Read the model definition and answer for the solid it produces. Units are mm, in the model's axes. A direction names the side the tool comes from. Give positions to 0.01 mm unless a question says otherwise; leave off trailing zeros. Loops run counter-clockwise (first coordinate to the right, second up) from the corner with the lowest first, then second, coordinate; pieces in that order, holes last. Notation, with made-up numbers: (61, 14) - (113, 14) arc R25 ccw to (113, 42) - close; hole circle Ø9 at (38, -8). An arc over 180 degrees is marked (long way). Write item = value, one per line. Start each with the question number.
from build123d import *

# Parameters (mm, degrees)
F1_DEPTH = 13.97
F3_D     = 4.7625
F4_W     = 19.05
F4_H     = 13.97
F5_DEPTH = 8.89
F7_D     = 4.7625


with BuildPart() as f1:
    # F0 (on Top) → F1 (new body)
    with BuildSketch(Plane.XY):
        with BuildLine():
            ThreePointArc((-30.457825, -6.426635), (-18.69401, -17.139455), (-7.62, -5.715))
            ThreePointArc((-7.62, -5.715), (-10.967769, 2.367231), (-19.05, 5.715))
            ThreePointArc((-19.05, 5.715), (-24.765, 4.18367), (-28.94867, 0))
            ThreePointArc((-28.94867, 0), (-30.177313, -3.101994), (-30.457825, -6.426635))
        make_face()
        with BuildLine():
            Line((-7.62, -5.715), (19.05, -5.715))
            Line((19.05, -5.715), (19.05, 5.715))
            Line((19.05, 5.715), (-19.05, 5.715))
            ThreePointArc((-19.05, 5.715), (-10.967769, 2.367231), (-7.62, -5.715))
        make_face()
        with BuildLine():
            Line((-32.65909, -6.426635), (-30.457825, -6.426635))
            ThreePointArc((-30.457825, -6.426635), (-30.177313, -3.101994), (-28.94867, 0))
            Line((-28.94867, 0), (-32.65909, -6.426635))
        make_face()
    extrude(amount=F1_DEPTH)

    # F3 (through all)
    with Locations(Plane.XY.offset(13.97)):
        with Locations((-19.05, -5.715)):
            Hole(F3_D / 2)

    # F4 (on face) → F5 (cut)
    with BuildSketch(Plane.XZ.offset(5.715)):
        with Locations((9.525, 6.985)):
            Rectangle(F4_W, F4_H)
    extrude(amount=-F5_DEPTH, mode=Mode.SUBTRACT)

    # F7 (through all)
    with Locations(Plane.XZ.offset(-3.175)):
        with Locations((14.605, 7.200924)):
            Hole(F7_D / 2)


solid = f1.part
1. A cutting plane is placed at D-D on y = 0.5. Give the vertices of the cut face in (x, z), and give its area (3 significant figures).
2. Given P1, Ø1.1, axis at x = -32, z = 6.5, coming from the -Y side; P2, Ø2, axis at y = -8, z = 7, coming from the +X side; P3, Ø4.5, axis at y = -1, z = 8, coming from the +X side; P4, Ø1, axis at x = 1.5, y = -7, coming from the -Z side, each flat-ended and moving along its own axis, determine where each tip first touches the part or whether it passes through.
3. A cutting plane is placed at C-C on x = -5. Give the vertices of the cut face in (y, z) (3 decimals).
4. A tool of negligible diameter and unlimited length cuts with its end or side. For faces 1 (the flat face through (-4, -5.715, 7)), 2 (the flat face through (-32, -6.427, 7)), 3 (the cylindrical face through (-21.32, -5, 6.89)), from which of +Z, -Z, +X, -X, +Y, -Y can it reach the whole face along a straight path? Write none if from no direction.
5. Consider line 1 along Y through (x, z) = (-19.05, 8.75) (3 decimals); line 2 along X through (y, z) = (4, 6.5); line 3 along Y through (x, z) = (1, 3.75) (3 decimals). Determine where each line is inside the solid, lowest interval first. Write a range as [from, to].
6. A cutting plane is placed at A-A on z = 6.5. Give the number of separate pieces and of enclosed holes in the cut face, and give its area (4 significant figures).
7. For a pull along Z with two mould halves and no side action, classify faces 4 (the cylindrical face through (16.495, 4.463, 5.752)), 5 (the flat face through (19.05, 4, 7)), 6 (the flat face through (-13, -3, 13.97)) as released by +Z, released by -Z, zero draft, split by the parting line, or undercut.
Reply:
q1.outline = (-28.64, 0) - (0, 0) - (0, 13.97) - (-28.64, 13.97) - close
q1.area = 400 mm^2
q2.P1 = -6.43
q2.P2 = -7.69
q2.P3 = 0
q2.P4 = through
q3.outline = (-5.715, 0) - (5.715, 0) - (5.715, 13.97) - (-5.715, 13.97) - close
q4.face_1 = +Z, -Z, +X, -Y
q4.face_2 = +Z, -Z, -X, -Y
q4.face_3 = +Z, -Z
q5.line_1 = [-17.145, -8.096], [-3.334, 5.715]
q5.line_2 = [-25.07, 12.33], [16.88, 19.05]
q5.line_3 = [3.175, 5.715]
q6.separate_pieces = 2
q6.enclosed_holes = 1
q6.area = 549.5 mm^2
q7.face_4 = undercut
q7.face_5 = zero draft
q7.face_6 = released by +Z
